```python
from build123d import *

# Parameters (mm, degrees)
F1_DEPTH = 3
F3_DEPTH = 3
F5_DEPTH = 3
F6_W     = 660
F6_H     = 944.517678
F7_DEPTH = 3
F8_DEPTH = 3


with BuildPart() as f1:
    # F0 (on Front) → F1 (new body)
    with BuildSketch(Plane.XZ):
        Polygon((-387, 1045), (-387, 165.699527), (-387, 5), (387, 5), (387, 165.699527), (387, 1045), (327, 1045), (327, 572.928839), (-327, 572.928839), (-327, 1045), align=None)
    extrude(amount=F1_DEPTH)

    # F2 (on face) → F3 (join)
    with BuildSketch(Plane(origin=(327, 0, 0), x_dir=(0, -1, 0), z_dir=(-1, 0, 0))):
        Polygon((820.651236, 1045), (0, 1045), (0, 572.928839), (3, 572.928839), align=None)
        Polygon((820.651236, 1045), (3, 1045), (3, 572.928839), align=None)
    extrude(amount=-F3_DEPTH)

    # F4 (on face) → F5 (join)
    with BuildSketch(Plane.YZ.offset(-327)):
        Polygon((0, 1045), (-3, 1045), (-820.651236, 1045), (-3, 572.928839), (0, 572.928839), align=None)
    extrude(amount=-F5_DEPTH)

    # F6 (on face) → F7 (join)
    with BuildSketch(Plane(origin=(0, 247.335464, 428.397591), x_dir=(1, 0, 0), z_dir=(0, -0.5, -0.866025))):
        with Locations((0, 760.945979)):
            Rectangle(F6_W, F6_H)
    extrude(amount=F7_DEPTH)

    # F6 (on face) → F8 (join)
    with BuildSketch(Plane(origin=(0, 247.335464, 428.397591), x_dir=(1, 0, 0), z_dir=(0, -0.5, -0.866025))):
        with Locations((0, 760.945979)):
            Rectangle(F6_W, F6_H)
    extrude(amount=F8_DEPTH)


solid = f1.part
```
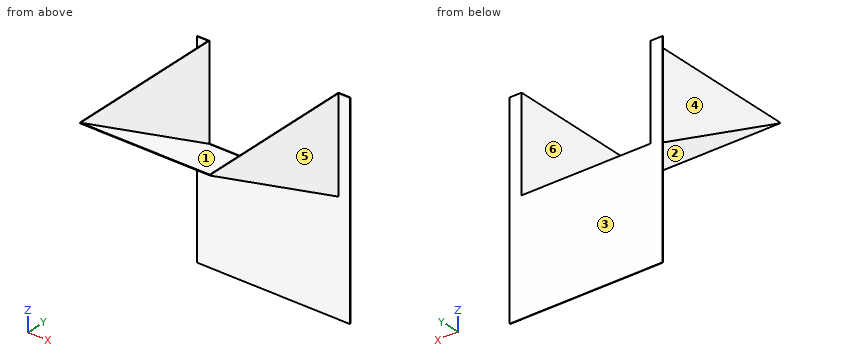
Geometry: final body of the model. Coordinates: model frame, mm. Face numbers are marked on the shaded views. A direction names the side the tool comes from. Give positions to 0.01 mm unless a question says otherwise; leave off trailing zeros. Order: outer loops, then holes, each group sorted by start corner. A loop starts at its lowest first (then second) coordinate and runs counter-clockwise, first axis right, second up. Notation, with made-up numbers: (60, 7) -> (116, 7) arc R26 cw to (116, 41) -> close; hole circle Ø8 at (7, -21). An arc over 180 degrees is marked (long way). Write each question's results on one line, items separated by ' | '. Start each with the question number.
1) Section A-A (x = -42.5). Return loops of the section in (y, z).
2) Section D-D (z = 765.5). Return loops of the section in (x, y).
3) Line query: line 1 (Y direction, x = 112, z = 84); line 2 (Z direction, x = 58, y = -626); line 3 (Z direction, x = -252, y = -764). Output: solid intervals per line, ascending. Write a range as from..to.
4) Set-up query: the marked faces 1 and 2. Return all of +Z, -Z, +X, -X, +Y, -Y with unobstructed straight access to the full face (end or side cutting, diameter ignored); none if empty.
5) Section B-B (y = -77.5). Return loops of the section in (x, z).
6) First-contact query: pin 1 (2 mm diameter, centred on x = -155, y = -559, fed in from -Z); pin 2 (2 mm diameter, centred on x = -141.5, y = -144.5, fed in from +Z); pin 3 (2 mm diameter, centred on y = -277.5, z = 924.5, fed in from -X). Flat tips, straight axial feed; report the tip coordinate or a pass-through.
7) Draft query along X for the marked faces 3, 4, 5 and 6. Return one class per face: pulls with the +X half, pulls with the -X half, needs draft (parallel to the pull), parting line crosses it, or undercut.
8) Section C-C (z = 610.5). Return loops of the section in (x, y), then the cut area to 3 significant figures.
Calculated:
1) outline: (-822.15, 1042.4) -> (-4.17, 570.14) -> (-3, 572.18) -> (-3, 5) -> (0, 5) -> (0, 572.93) -> (-3, 572.93) -> (-820.65, 1045) -> close
2) outline: (-387, -3) -> (-330, -3) -> (-330, -342.54) -> (330, -342.54) -> (330, -3) -> (387, -3) -> (387, 0) -> (327, 0) -> (327, -336.54) -> (-327, -336.54) -> (-327, 0) -> (-387, 0) -> close
3) line 1: -3..0 | line 2: 929.15..932.62 | line 3: 1008.83..1012.29
4) face 1: +Z, +Y | face 2: -Z, +X, -X, -Y
5) outline: (-330, 612.48) -> (330, 612.48) -> (330, 1045) -> (327, 1045) -> (327, 615.94) -> (-327, 615.94) -> (-327, 1045) -> (-330, 1045) -> close
6) pin 1: z = 889.89 | pin 2: z = 655.2 | pin 3: x = -330
7) face 3: needs draft | face 4: pulls with the -X half | face 5: pulls with the +X half | face 6: undercut
8) outline: (-387, -3) -> (-330, -3) -> (-330, -74.08) -> (330, -74.08) -> (330, -3) -> (387, -3) -> (387, 0) -> (327, 0) -> (327, -68.08) -> (-327, -68.08) -> (-327, 0) -> (-387, 0) -> close | area: 4,710 mm2
